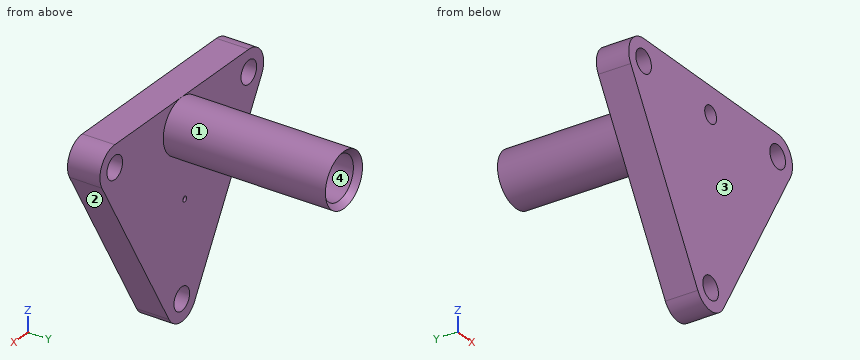
from build123d import *

# Parameters (mm, degrees)
SKETCH1_R           = 1.054
BOSS_EXTRUDE1_DEPTH = 3
SKETCH2_R           = 0.8
CUT_EXTRUDE1_DEPTH  = 23.736281859
SKETCH3_R           = 2.5
BOSS_EXTRUDE2_DEPTH = 15
CUT_EXTRUDE2_REACH  = 29.073
SKETCH4_R           = 2
CHAMFER1_SIZE       = 2
CHAMFER1_SIZE2      = 0.727940469
CHAMFER2_SIZE       = 0.5
SKETCH5_R           = 0.25
CUT_EXTRUDE3_DEPTH  = 0.25


with BuildPart() as part:
    # Sketch1 → Boss-Extrude1 (new body)
    with BuildSketch(Plane(origin=(0, 0, 0), x_dir=(1, 0, 0), z_dir=(0, 1, 0))):
        with BuildLine():
            Line((0, 0), (9.035898385, 0))
            ThreePointArc((9.035898385, 0), (10.767949192, 1), (10.767949192, 3))
            Line((10.767949192, 3), (1.732050808, 18.650635095))
            ThreePointArc((1.732050808, 18.650635095), (0, 19.650635095), (-1.732050808, 18.650635095))
            Line((-1.732050808, 18.650635095), (-10.767949192, 3))
            ThreePointArc((-10.767949192, 3), (-10.767949192, 1), (-9.035898385, 0))
            Line((-9.035898385, 0), (0, 0))
        make_face()
        with Locations(Location((0, 17.650635095, 0), (0, 0, 270))):
            Circle(SKETCH1_R, mode=Mode.SUBTRACT)
        with Locations(Location((-9.035898385, 2, 0), (0, 0, 270))):
            Circle(SKETCH1_R, mode=Mode.SUBTRACT)
        with Locations(Location((9.035898385, 2, 0), (0, 0, 270))):
            Circle(SKETCH1_R, mode=Mode.SUBTRACT)
    extrude(amount=BOSS_EXTRUDE1_DEPTH)

    # Sketch2 → Cut-Extrude1 (cut, through all)
    with BuildSketch(Plane(origin=(0, 3, 0), x_dir=(1, 0, 0), z_dir=(0, 1, 0))):
        with Locations(Location((0, 2.5, 0), (0, 0, 270))):
            Circle(SKETCH2_R)
    extrude(amount=-CUT_EXTRUDE1_DEPTH, mode=Mode.SUBTRACT)

    # Sketch3 → Boss-Extrude2 (add)
    with BuildSketch(Plane(origin=(0, 3, 0), x_dir=(1, 0, 0), z_dir=(0, 1, 0))):
        with Locations(Location((0, 2.5, 0), (0, 0, 270))):
            Circle(SKETCH3_R)
    extrude(amount=BOSS_EXTRUDE2_DEPTH)

    # Sketch4 → Cut-Extrude2 (cut, up to next)
    with BuildSketch(Plane(origin=(0, 3, 0), x_dir=(1, 0, 0), z_dir=(0, 1, 0)), mode=Mode.PRIVATE) as cut_extrude2_sk1:
        with Locations(Location((0, 2.5, 0), (0, 0, 270))):
            Circle(SKETCH4_R)
    cut_extrude2_tool1 = extrude(cut_extrude2_sk1.sketch, amount=CUT_EXTRUDE2_REACH, mode=Mode.PRIVATE) & part.part
    add(cut_extrude2_tool1.solids().sort_by_distance((0, 3, -2.5))[0], mode=Mode.SUBTRACT)

    # Chamfer1
    chamfer1_edges = [part.edges().sort_by_distance(p)[0] for p in [
        (0, 3, -4.5),
    ]]
    chamfer1_side = [part.faces().sort_by_distance(p)[0] for p in [
        (0, 10.5, -4.5),
    ]]
    chamfer(chamfer1_edges, length=CHAMFER1_SIZE, length2=CHAMFER1_SIZE2, reference=chamfer1_side[0])

    # Chamfer2
    chamfer2_edges = [part.edges().sort_by_distance(p)[0] for p in [
        (0, 18, -4.5),
    ]]
    chamfer(chamfer2_edges, length=CHAMFER2_SIZE - 0.0001)  # a hair under: the kernel refuses the full size

    # Sketch5 → Cut-Extrude3 (cut)
    with BuildSketch(Plane(origin=(0, 3, 0), x_dir=(1, 0, 0), z_dir=(0, 1, 0))):
        with Locations(Location((-0.400704282, 9.113083691, 0), (0, 0, 270))):
            Circle(SKETCH5_R)
    extrude(amount=-CUT_EXTRUDE3_DEPTH, mode=Mode.SUBTRACT)


solid = part.part
The listing builds one solid part. Answer for the finished solid, in the listing's coordinates (mm). Face numbers are marked on the shaded views. Give positions to 0.01 mm unless a question says otherwise; leave off trailing zeros. Write each loop counter-clockwise with the first axis right and the second up, starting at its lowest first coordinate (ties: lowest second). Pieces come first, ordered by that corner, then holes.
Item 1: Section D-D, the plane x = -7.5 is taken. Write down the section's boundary in (y, z), plus the area to 3 significant figures.
Item 2: Find the intervals of material crossed by line 1 along X through (y, z) = (0.85, -2.5); line 2 along X through (y, z) = (12.75, -2.5); line 3 along Z through (x, y) = (0.5, 1), in increasing order.
Item 3: Section C-C, the plane z = -2.5 is taken. Count the separate pieces of the cut face and the enclosed holes in it, plus the area to 3 significant figures.
Item 4: Flat-ended cylindrical pins translate along their axes: P1, Ø4, axis at x = 8, z = -5.5, coming from the +Y side; P2, Ø1.5, axis at y = 4.5, z = -14.5, coming from the +X side; P3, Ø3, axis at x = -0.5, z = -3, coming from the +Y side; P4, Ø1, axis at y = 2.5, z = -17.5, coming from the +X side. Find the tip coordinate at first contact, or state that the pin passes through.
Item 5: Section B-B, the plane y = 9 is taken. Write down the section's boundary in (x, z), plus the area to 3 significant figures.
Item 6: Section A-A, the plane z = -17 is taken. Write down the section's boundary in (x, y), plus the area to 3 significant figures.
Item 7: Determine the mould class of the marked faces 1, 2, 3 and 4 for opening direction X: released by +X, released by -X, zero draft, split by the parting line, or undercut.
Completed:
1. outline: (0, -8.66) - (3, -8.66) - (3, 0) - (0, 0) - close
1. area: 26.0 mm2
2. line 1: x = -10.97 to -9.96, -8.11 to -0.8, 0.8 to 8.11, 9.96 to 10.97
2. line 2: x = -2.5 to -2, 2 to 2.5
2. line 3: z = -19.59 to -18.58, -16.72 to -3.12, -1.88 to 0
3. separate pieces: 4
3. enclosed holes: 0
3. area: 66.1 mm2
4. P1: stops at y = 3
4. P2: passes through
4. P3: stops at y = 17.71
4. P4: stops at x = 2.69
5. outline: circle Ø5 at (0, -2.5); hole circle Ø4 at (0, -2.5)
5. area: 7.07 mm2
6. outline: (-2.69, 0) - (-0.83, 0) - (-0.83, 3) - (-2.69, 3) - close; (0.83, 0) - (2.69, 0) - (2.69, 3) - (0.83, 3) - close
6. area: 11.1 mm2
7. face 1: split by the parting line
7. face 2: released by +X
7. face 3: zero draft
7. face 4: undercut
